Autodesk Inventor part; units mm, degrees
ref_plane "YZ Plane" through (0, 0, 0) normal (1, 0, 0) x (0, 1, 0)
ref_plane "XZ Plane" through (0, 0, 0) normal (0, 1, 0) x (-1, 0, 0)
ref_plane "XY Plane" through (0, 0, 0) normal (0, 0, 1) x (1, 0, 0)
sketch "Sketch1" plane through (0, 0, 0) normal (0, 0, 1) x (1, 0, 0)
  arc A0 (0, 14.224) -> (0, -14.224) centre (0, 0) ccw construction
  arc A1 (0, 17.4307) -> (0, -17.4308) centre (0, 0) ccw
  line L0 (0, 0) -> (-25.4, 0)
  circle A2 centre (-25.4, 0) radius 4.7625 construction
  line L1 (0, 14.224) -> (0, -14.224)
  circle A3 centre (-25.4, 0) radius 7.9692
  line L2 (0, 14.224) -> (0, 17.4307)
  line L3 (0, -14.224) -> (0, -17.4308)
  line L4 (-28.3685, 7.3957) -> (-6.493, 16.1763)
  line L5 (-28.3685, -7.3957) -> (-6.493, -16.1763)
  point P0 (-11.176, 0)
  dimension "d0" = 28.448
  dimension "d2" = 25.4
  dimension "d3" = 9.525
  dimension "d6" = 3.2067
  dimension "d7" = 3.2067
  dimension "d8" = 11.176
extrude "Extrusion1" add sketch "Sketch1" along normal blind 4.7625
hole "Hole1" at (-25.4, 0, 0) direction (0, 0, 1) diameter 4.9784 end through all
hole "Hole2" at (-11.176, 0, 0) direction (0, 0, 1) diameter 4.2164 end through all
mirror "Mirror1" about plane through (0, -17.4308, 0) normal (1, 0, 0)
equation "\"d6\" = d7"
properties part number "Pneumatic Mounting Plate"
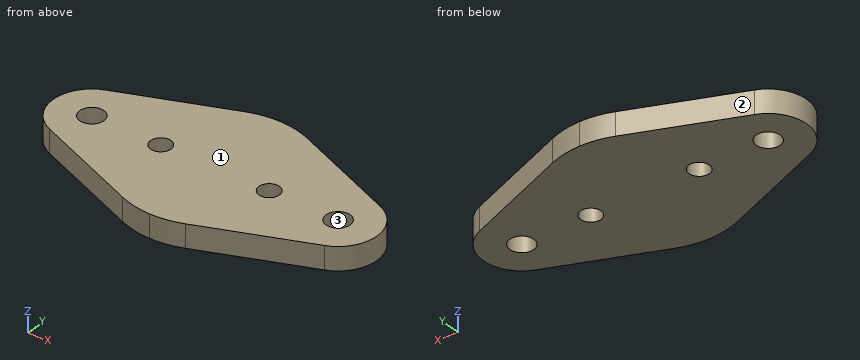
Input: part model. Units: mm. Frame: model coordinates. Face numbers are marked on the shaded views. Coordinates: 2 decimals unless noted, no trailing zeros. Loops run counter-clockwise (first coordinate to the right, second up) from the corner with the lowest first, then second, coordinate; pieces in that order, holes last. Notation, with made-up numbers: (87.25, 13) - (116.25, 13) arc R24 cw to (116.25, 51) - close; hole circle Ø6 at (48.25, -14). An arc over 180 degrees is marked (long way). Answer in a Markdown table with one row per item. Add a question column.
Item 1: Section query C-C on z = 3.3. Return the cut outline in (x, y).
Item 2: Section query B-B on x = 25.4. Return the cut outline in (y, z), then the cut area to 3 significant figures.
Item 3: Contact query for flat-ended pins moving along their axis: P1, Ø1, axis at x = -21.5, z = 4, coming from the +Y side; P2, Ø1.5, axis at x = -10, z = 1, coming from the -Y side; P3, Ø4.5, axis at x = 25.4, y = 0, coming from the +Z side. Output: stop coordinate, or through.
Item 4: Line query: line 1 along Y through (x, z) = (-11, 1.4); line 2 along Y through (x, z) = (-25.4, 1.65); line 3 along Y through (x, z) = (-0.5, 2.6). Output: solid intervals per line, ascending. Write a range as [from, to].
Item 5: Section query D-D on x = 12. Return the cut outline in (y, z), then the cut area to 3 significant figures.
Item 6: Section query A-A on y = 0. Return the cut outline in (x, z), then the cut area to 3 significant figures.
Item 7: Mould query, pull axis X, two halves, no side actions, for the marked faces 1, 2 and 3. Classes: released by +X, released by -X, zero draft, split by the parting line, or undercut.
Recorded:
| question | item | result |
|---|---|---|
| 1 | outline | (-28.37, -7.4) - (-6.49, -16.18) arc R17.43 ccw to (0, -17.43) arc R17.43 ccw to (6.49, -16.18) - (28.37, -7.4) arc R7.97 ccw to (28.37, 7.4) - (6.49, 16.18) arc R17.43 ccw to (0, 17.43) arc R17.43 ccw to (-6.49, 16.18) - (-28.37, 7.4) arc R7.97 ccw to start; hole circle Ø4.98 at (-25.4, 0); hole circle Ø4.22 at (-11.18, 0); hole circle Ø4.22 at (11.18, 0); hole circle Ø4.98 at (25.4, 0) |
| 2 | outline | (-8.59, 0) - (-2.49, 0) - (-2.49, 4.76) - (-8.59, 4.76) - close; (2.49, 0) - (8.59, 0) - (8.59, 4.76) - (2.49, 4.76) - close |
| 2 | area | 58.1 mm^2 |
| 3 | P1 | y = 10.35 |
| 3 | P2 | y = -15.07 |
| 3 | P3 | through |
| 4 | line 1 | [-14.37, -2.1], [2.1, 14.37] |
| 4 | line 2 | [-8.59, -2.49], [2.49, 8.59] |
| 4 | line 3 | [-17.42, 17.42] |
| 5 | outline | (-13.97, 0) - (-1.94, 0) - (-1.94, 4.76) - (-13.97, 4.76) - close; (1.94, 0) - (13.97, 0) - (13.97, 4.76) - (1.94, 4.76) - close |
| 5 | area | 115 mm^2 |
| 6 | outline | (-33.37, 0) - (-27.89, 0) - (-27.89, 4.76) - (-33.37, 4.76) - close; (-22.91, 0) - (-13.28, 0) - (-13.28, 4.76) - (-22.91, 4.76) - close; (-9.07, 0) - (9.07, 0) - (9.07, 4.76) - (-9.07, 4.76) - close; (13.28, 0) - (22.91, 0) - (22.91, 4.76) - (13.28, 4.76) - close; (27.89, 0) - (33.37, 0) - (33.37, 4.76) - (27.89, 4.76) - close |
| 6 | area | 230 mm^2 |
| 7 | face 1 | zero draft |
| 7 | face 2 | released by -X |
| 7 | face 3 | undercut |
